The listing builds one solid part. Answer for the finished solid, in the listing's coordinates (mm). A direction names the side the tool comes from. Round coordinates to 2 decimals unless told otherwise and drop trailing zeros. Order: outer loops, then holes, each group sorted by start corner. A loop starts at its lowest first (then second) coordinate and runs counter-clockwise, first axis right, second up. Notation, with made-up numbers: (-34.5, -38.75) - (-17.5, -38.75) arc R24 cw to (-17.5, -16.75) - close; hole circle Ø3 at (-36.75, -17.75). An arc over 180 degrees is marked (long way). Use CSV: the item, a comma, the result in double quotes. Start each with the question number.
Item 1: Find section A-A, the plane y = -9. Give the vertices of the cut face in (x, z).
Item 2: Straight lines are drawn through the part: line 1 along X through (y, z) = (8.5, 7.5); line 2 along Z through (x, y) = (16, 4.75); line 3 along Z through (x, y) = (9, 11). For each, find the intervals that lie inside material, in ascending order. Write a range as [from, to].
Item 3: Flat-ended cylindrical pins translate along their axes: P1, Ø2.5, axis at x = 17.5, y = -4, coming from the +Z side; P2, Ø1.5, axis at x = -8, y = -0.5, coming from the +Z side; P3, Ø1.6, axis at x = 6.5, z = 6.5, coming from the -Y side. Find the tip coordinate at first contact, or state that the pin passes through.
Item 4: Find section C-C, the plane z = 6.25. Count the separate pieces of the cut face and the enclosed holes in it, plus the area to 3 significant figures.
Item 5: Determine the mould class of faces 6 (the flat face through (7, -10, 7)), 7 (the flat face through (9.617, -10, 6)), 8 (the flat face through (-2.334, 0, 9)) for opening direction X: +X half, -X half, draft (parallel to the pull), parting line (faces both ways), or undercut.
Item 6: Find section D-D, the plane x = 20. Give the vertices of the cut face in (y, z).
Item 7: For faces 1 (the flat face through (0.814, -10, 6)), 2 (the cylindrical face through (5.05, 11.74, 7.46)), 3 (the flat face through (-2, -11.72, 6)), 4 (the flat face through (-5.733, 0, 7)), 5 (the flat face through (7, -8.132, 6)), determine the directions among +Z, -Z, +X, -X, +Y, -Y from which every point of the face is accessible in a straight line to the end or side of a thin tool.
Item 8: Find section B-B, the plane x = -11. Give the vertices of the cut face in (y, z), plus the area to 3 significant figures.
```python
from build123d import *

# Parameters (mm, degrees)
SKETCH_1_W      = 45
SKETCH_1_H      = 26
EXTRUDE_1_DEPTH = 5
SKETCH_2_R      = 6
EXTRUDE_2_DEPTH = 26
SKETCH_3_W      = 14
SKETCH_3_H      = 14
EXTRUDE_3_DEPTH = 8
SKETCH_4_R      = 2.5
EXTRUDE_4_DEPTH = 5
SKETCH_5_W      = 11
SKETCH_5_H      = 11
EXTRUDE_5_DEPTH = 4
SKETCH_6_W      = 6.186657106
SKETCH_6_H      = 3.588261122
SKETCH_6_W_2    = 6.062923964
EXTRUDE_6_DEPTH = 2
SKETCH_7_W      = 11.669170616
SKETCH_7_H      = 6.291205027
EXTRUDE_7_DEPTH = 3


with BuildPart() as part:
    # Эскиз1 → Бобышка-Вытянуть1 (new body)
    with BuildSketch(Plane.XY):
        Rectangle(SKETCH_1_W, SKETCH_1_H)
    extrude(amount=EXTRUDE_1_DEPTH)

    # Эскиз2 → Бобышка-Вытянуть2 (add)
    with BuildSketch(Plane(origin=(0, 13, 0), x_dir=(1, 0, 0), z_dir=(0, 1, 0))):
        with Locations((-27.954356057, -2.5)):
            Circle(SKETCH_2_R)
    extrude(amount=-EXTRUDE_2_DEPTH)

    # Эскиз3 → Бобышка-Вытянуть3 (add)
    with BuildSketch(Plane.XY.offset(5)):
        with Locations((4.666405911, 0)):
            Rectangle(SKETCH_3_W, SKETCH_3_H)
    extrude(amount=EXTRUDE_3_DEPTH)

    # Эскиз4 → Бобышка-Вытянуть4 (add)
    with BuildSketch(Plane.XY.offset(5)):
        with Locations((-1.458384625, 10.053317798)):
            Circle(SKETCH_4_R)
        with Locations((6.893602469, 10.053317798)):
            Circle(SKETCH_4_R)
        with Locations((16.854120411, -4.9183924)):
            Circle(SKETCH_4_R)
    extrude(amount=EXTRUDE_4_DEPTH)

    # Эскиз5 → Бобышка-Вытянуть5 (add)
    with BuildSketch(Plane.XY.offset(5)):
        with Locations((-11.233302854, 0)):
            Rectangle(SKETCH_5_W, SKETCH_5_H)
    extrude(amount=EXTRUDE_5_DEPTH)

    # Эскиз6 → Бобышка-Вытянуть6 (add)
    with BuildSketch(Plane.XY.offset(5)):
        with Locations((-2.279728316, -9.926144411)):
            Rectangle(SKETCH_6_W, SKETCH_6_H)
        with Locations((6.585206892, -9.926144411)):
            Rectangle(SKETCH_6_W_2, SKETCH_6_H)
    extrude(amount=EXTRUDE_6_DEPTH)

    # Эскиз7 → Бобышка-Вытянуть7 (add)
    with BuildSketch(Plane.XY.offset(5)):
        with Locations((23.730450038, 7.608351051)):
            Rectangle(SKETCH_7_W, SKETCH_7_H)
    extrude(amount=EXTRUDE_7_DEPTH)


solid = part.part
```
Worked out:
1,outline,"(-22.5, 0) - (22.5, 0) - (22.5, 5) - (9.62, 5) - (9.62, 7) - (3.55, 7) - (3.55, 5) - (0.81, 5) - (0.81, 7) - (-5.37, 7) - (-5.37, 5) - (-22.5, 5) arc R6 ccw (long way) to start"
2,line 1,"x = [-31.27, -24.64], [-3.42, 0.5], [4.93, 8.85], [17.9, 29.57]"
2,line 2,"z = [0, 5]"
2,line 3,"z = [0, 10]"
3,P1,"stops at z = 10"
3,P2,"stops at z = 9"
3,P3,"stops at y = -11.72"
4,separate pieces,"9"
4,enclosed holes,"0"
4,area,"737 mm²"
5,face 6,"draft"
5,face 7,"+X half"
5,face 8,"undercut"
6,outline,"(-13, 0) - (13, 0) - (13, 5) - (10.75, 5) - (10.75, 8) - (4.46, 8) - (4.46, 5) - (-13, 5) - close"
7,face 1,"+Z, -Y"
7,face 2,"+Z"
7,face 3,"+Z, +X, -Y"
7,face 4,"+Z, +Y, -Y"
7,face 5,"+Z, +X"
8,outline,"(-13, 0) - (13, 0) - (13, 5) - (5.5, 5) - (5.5, 9) - (-5.5, 9) - (-5.5, 5) - (-13, 5) - close"
8,area,"174 mm²"
